Job drawing, mm, ordinate dimensions from the low corner. One solid piece. Round coordinates to 2 decimals unless told otherwise and drop trailing zeros. Loops run counter-clockwise (first coordinate to the right, second up) from the corner with the lowest first, then second, coordinate; pieces in that order, holes last.
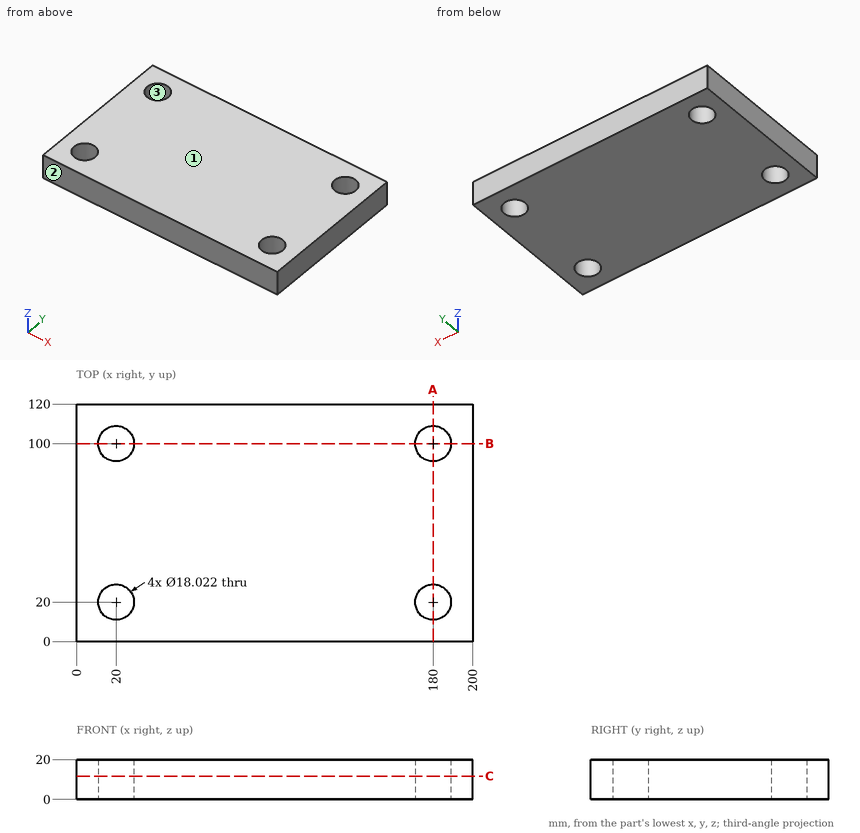
(1) Slice it at B-B on y = 100. List the corners of the cut face in (x, z).
Responses:
outline: (0, 0) - (10.99, 0) - (10.99, 20) - (0, 20) - close; (29.01, 0) - (170.99, 0) - (170.99, 20) - (29.01, 20) - close; (189.01, 0) - (200, 0) - (200, 20) - (189.01, 20) - close
(2) Slice it at C-C on z = 11.75. List the corners of the cut face in (x, y), plus the area to 3 significant figures.
Responses:
outline: (0, 0) - (200, 0) - (200, 120) - (0, 120) - close; hole circle Ø18.02 at (20, 20); hole circle Ø18.02 at (20, 100); hole circle Ø18.02 at (180, 20); hole circle Ø18.02 at (180, 100)
area: 23,000 mm2
(3) Pin check, flat tip, straight feed: P1, Ø3, axis at x = 39, y = 57, coming from the -Z side. Stop position of the tip, or through.
Responses:
P1: stops at z = 0
(4) Slice it at A-A on x = 180. List the corners of the cut face in (y, z).
Responses:
outline: (0, 0) - (10.99, 0) - (10.99, 20) - (0, 20) - close; (29.01, 0) - (90.99, 0) - (90.99, 20) - (29.01, 20) - close; (109.01, 0) - (120, 0) - (120, 20) - (109.01, 20) - close
(5) Probe line 1 (X direction, y = 20, z = 15.25); line 2 (Y direction, x = 180, z = 6); line 3 (X direction, y = 94, z = 6.25). List the from-to ranges inside material, lowest first.
Responses:
line 1: x = 0 to 10.99, 29.01 to 170.99, 189.01 to 200
line 2: y = 0 to 10.99, 29.01 to 90.99, 109.01 to 120
line 3: x = 0 to 13.28, 26.72 to 173.28, 186.72 to 200
(6) Pull direction Y, two halves, no side cores. Call the marked faces 1, 2 and 3: +Y half, -Y half, draft (parallel to the pull), parting line (faces both ways), or undercut.
Responses:
face 1: draft
face 2: -Y half
face 3: undercut
